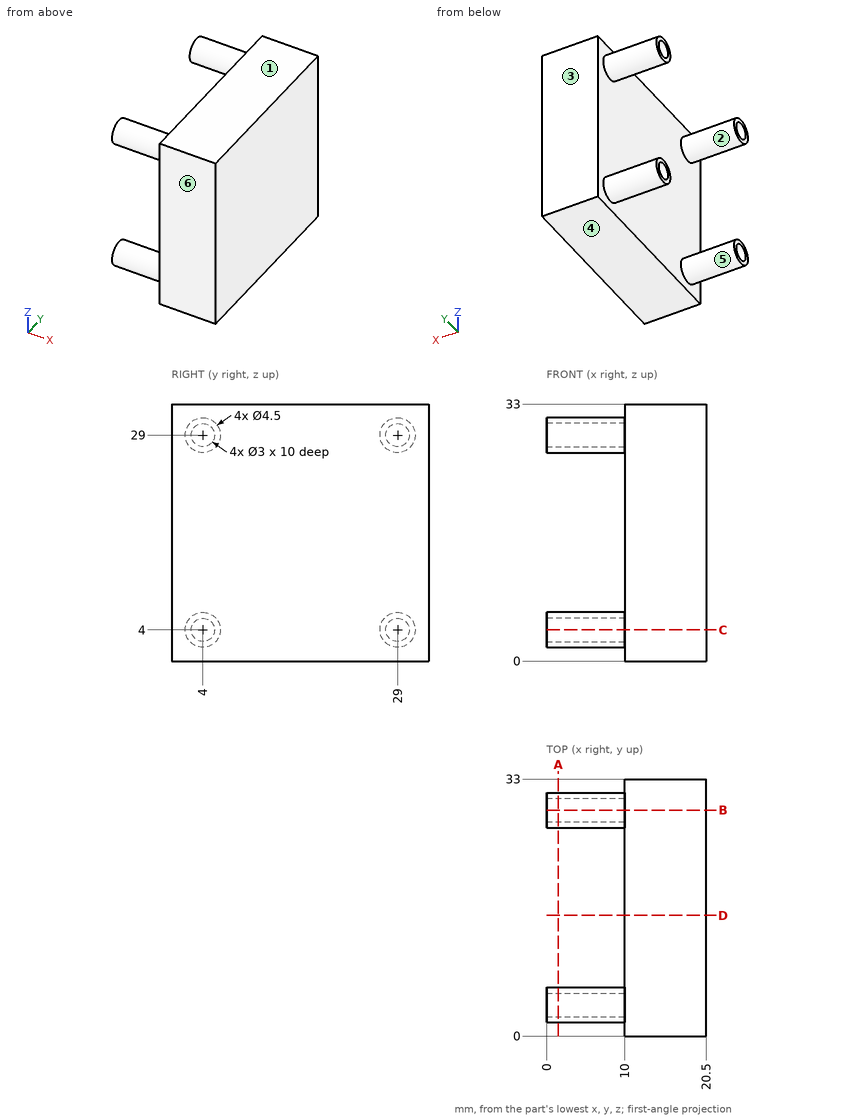
The drawing under review shows one solid part. Ordinate dimensions are in mm from its lowest x, y, z. A direction names the side the tool comes from. Coordinates: 2 decimals unless noted, no trailing zeros. Loops run counter-clockwise (first coordinate to the right, second up) from the corner with the lowest first, then second, coordinate; pieces in that order, holes last. Notation, with made-up numbers: (70.25, 56.5) - (100.25, 56.5) arc R24 ccw to (100.25, 88.5) - close; hole circle Ø4 at (39.25, 85.5). An arc over 180 degrees is marked (long way). Use CSV: the item, a comma, the result in double quotes. Start each with the question number.
1. Add section D-D on y = 15.5. Give the boundary of the cut face in (x, z).
2. Mouldability with a two-part tool opening along Z and no side actions: class the marked faces 1, 2, 3 and 4 as released by +Z, released by -Z, zero draft, split by the parting line, or undercut.
3. Add section A-A on x = 1.5. Give the boundary of the cut face in (y, z), plus the area to 3 significant figures.
4. For the marked faces 5 and 6, list the 3-axis set-ups (+Z, -Z, +X, -X, +Y, -Y) from which the entire face can be reached by the end or side of a thin tool; tool diameter is ignored.
5. Add section B-B on y = 29. Give the boundary of the cut face in (x, z).
6. Clearance check with flat-ended pins moving along their axes: pin 1 (2.5 mm diameter, centred on y = 4, z = 29, fed in from -X); pin 2 (4 mm diameter, centred on x = 7, z = 9.5, fed in from -Y). State where each tip first meets the part, or that it passes through.
7. To check wall thickness, follow probe 1 along Y at (x, z) = (2.75, 29); probe 2 along Z at (x, y) = (5.75, 3). State the ranges of each line that lie inside material, in increasing order.
Resolved:
1,outline,"(10, 0) - (20.5, 0) - (20.5, 33) - (10, 33) - close"
2,face 1,"released by +Z"
2,face 2,"undercut"
2,face 3,"zero draft"
2,face 4,"released by -Z"
3,outline,"circle Ø4.5 at (4, 4); circle Ø4.5 at (4, 29); circle Ø4.5 at (29, 4); circle Ø4.5 at (29, 29); hole circle Ø3 at (4, 4); hole circle Ø3 at (4, 29); hole circle Ø3 at (29, 4); hole circle Ø3 at (29, 29)"
3,area,"35.3 mm2"
4,face 5,"-X"
4,face 6,"+Z, -Z, +X, -X, -Y"
5,outline,"(0, 1.75) - (10, 1.75) - (10, 0) - (20.5, 0) - (20.5, 33) - (10, 33) - (10, 31.25) - (0, 31.25) - (0, 30.5) - (10, 30.5) - (10, 27.5) - (0, 27.5) - (0, 26.75) - (10, 26.75) - (10, 6.25) - (0, 6.25) - (0, 5.5) - (10, 5.5) - (10, 2.5) - (0, 2.5) - close"
6,pin 1,"x = 10"
6,pin 2,"through"
7,probe 1,"1.75 to 2.5, 5.5 to 6.25, 26.75 to 27.5, 30.5 to 31.25"
7,probe 2,"1.98 to 2.88, 5.12 to 6.02, 26.98 to 27.88, 30.12 to 31.02"
